Geometry check sheet. Reference: the model listing, model coordinates, mm. A direction names the side the tool comes from. Coordinates: 2 decimals unless noted, no trailing zeros. Loops run counter-clockwise (first coordinate to the right, second up) from the corner with the lowest first, then second, coordinate; pieces in that order, holes last.
Autodesk Inventor part; units mm, degrees
ref_plane "YZ Plane" through (0, 0, 0) normal (1, 0, 0) x (0, 1, 0)
ref_plane "XZ Plane" through (0, 0, 0) normal (0, 1, 0) x (-1, 0, 0)
ref_plane "XY Plane" through (0, 0, 0) normal (0, 0, 1) x (1, 0, 0)
sketch "Boceto2" plane through (0, 0, 0) normal (0, 1, 0) x (-1, 0, 0)
  line L0 (0, 0) -> (100, 0)
  line L1 (100, 0) -> (100, -200)
  line L2 (100, -200) -> (0, -200)
  line L3 (0, -200) -> (0, 0)
  dimension "d2" = 200
  dimension "d3" = 100
extrude "Extrusión1" add sketch "Boceto2" along normal blind 5
sketch "Boceto3" plane through (0, 5, 0) normal (0, 1, 0) x (1, 0, 0)
  line L0 (-100, 200) -> (-100, 0)
  line L1 (-100, 55) -> (-120, 55)
  line L2 (-120, 55) -> (-120, 95)
  line L3 (-120, 95) -> (-100, 95)
  line L4 (-100, 95) -> (-100, 55)
  line L5 (0, 0) -> (0, 200)
  line L6 (0, 55) -> (20, 55)
  line L7 (20, 55) -> (20, 95)
  line L8 (20, 95) -> (0, 95)
  line L9 (0, 95) -> (0, 55)
  line L10 (-100, 0) -> (0, 0)
  circle A0 centre (-110, 75) radius 2.5
  circle A1 centre (10, 75) radius 2.5
  point P0 (0, 95)
  dimension "d6" = 20
  dimension "d7" = 40
  dimension "d8" = 20
  dimension "d9" = 40
  dimension "d10" = 55
  dimension "d11" = 5
  dimension "d12" = 5
extrude "Extrusión2" add sketch "Boceto3" against normal blind 5
thread "Rosca1"
thread "Rosca2"
sketch "Boceto4" plane through (0, 5, 0) normal (0, 1, 0) x (1, 0, 0)
  line L0 (-100, 200) -> (-100, 95)
  line L1 (0, 95) -> (0, 200)
  line L2 (-100, 200) -> (0, 200)
  line L3 (0, 200) -> (0, 190)
  line L4 (0, 190) -> (-100, 190)
  line L5 (-100, 190) -> (-100, 200)
  line L6 (0, 55) -> (-100, 55)
  line L7 (-100, 55) -> (-100, 65)
  line L8 (-100, 65) -> (0, 65)
  line L9 (0, 65) -> (0, 55)
  line L10 (-100, 15) -> (0, 15)
  line L11 (0, 15) -> (0, 25)
  line L12 (0, 25) -> (-100, 25)
  line L13 (-100, 25) -> (-100, 15)
  line L14 (-100, 0) -> (0, 0)
  dimension "d19" = 10
  dimension "d20" = 100
  dimension "d21" = 10
  dimension "d22" = 100
  dimension "d24" = 30
  dimension "d56" = 125
extrude "Extrusión3" add sketch "Boceto4" along normal blind 60
sketch "Boceto5" plane through (0, 0, -200) normal (0, 0, -1) x (-1, 0, 0)
  circle A0 centre (50, 40) radius 5
  line L0 (0, 0) -> (0, 65)
  line L1 (0, 0) -> (100, 0)
  dimension "d28" = 10
  dimension "d29" = 50
  dimension "d34" = 40
extrude "Extrusión4" cut sketch "Boceto5" against normal blind 10
sketch "Boceto6" plane through (0, 5, -65) normal (0, 0, -1) x (-1, 0, 0)
  circle A0 centre (50, 35) radius 5
  circle A1 centre (50, 35) radius 5
  point P0 (0, -5)
extrude "Extrusión5" cut sketch "Boceto6" against normal blind 10
sketch "Boceto7" plane through (-100, 5, -15) normal (0, 0, 1) x (1, 0, 0)
  circle A0 centre (50, 35) radius 5
  circle A1 centre (50, 35) radius 4
  circle A2 centre (36.1091, 50) radius 2.5
  circle A3 centre (63.8909, 50) radius 2.5
  line L0 (0, 0) -> (0, 60)
  line L1 (100, 0) -> (100, 60)
  circle A4 centre (34.6472, 21.5) radius 2.5
  circle A5 centre (65.3528, 21.5) radius 2.5
  line L2 (0, 60) -> (100, 60)
  line L3 (0, 0) -> (100, 0)
  point P0 (100, -5)
  dimension "d35" = 8
  dimension "d36" = 5
  dimension "d37" = 5
  dimension "d41" = 5
  dimension "d42" = 5
  dimension "d45" = 10
  dimension "d47" = 10
  dimension "d50" = 20.444
  dimension "d51" = 28.5
  dimension "d52" = 20.444
  dimension "d53" = 20.444
  dimension "d54" = 20.444
  dimension "d55" = 28.5
extrude "Extrusión6" cut sketch "Boceto7" against normal blind 10 contours A1 | A2 | A3 | A4 | A5
properties part number "Base_motor"
1) Section check D-D on y = 26.5. Record the cut outline in (x, z), and give its area (3 significant figures).
Data:
outline: (-100, -200) - (0, -200) - (0, -190) - (-100, -190) - close; (-100, -65) - (0, -65) - (0, -55) - (-100, -55) - close; (-100, -25) - (-67.85, -25) - (-67.85, -15) - (-100, -15) - close; (-62.85, -25) - (-37.15, -25) - (-37.15, -15) - (-62.85, -15) - close; (-32.15, -25) - (0, -25) - (0, -15) - (-32.15, -15) - close
area: 2,900 mm2
2) Section check C-C on x = 10. Record the cut outline in (y, z).
Data:
outline: (0, -95) - (5, -95) - (5, -77.5) - (0, -77.5) - close; (0, -72.5) - (5, -72.5) - (5, -55) - (0, -55) - close
3) Section check B-B on z = -75. Record the cut outline in (x, y), and give its area (3 significant figures).
Data:
outline: (-120, 0) - (-112.5, 0) - (-112.5, 5) - (-120, 5) - close; (-107.5, 0) - (7.5, 0) - (7.5, 5) - (-107.5, 5) - close; (12.5, 0) - (20, 0) - (20, 5) - (12.5, 5) - close
area: 650 mm2
4) Section check A-A on x = -50. Record the cut outline in (y, z).
Data:
outline: (0, -200) - (35, -200) - (35, -190) - (5, -190) - (5, -65) - (35, -65) - (35, -55) - (5, -55) - (5, -25) - (36, -25) - (36, -15) - (5, -15) - (5, 0) - (0, 0) - close; (44, -25) - (65, -25) - (65, -15) - (44, -15) - close; (45, -200) - (65, -200) - (65, -190) - (45, -190) - close; (45, -65) - (65, -65) - (65, -55) - (45, -55) - close
5) Mould release check, pull along Z, two halves, no side actions. Record for faces 1 (the flat face through (10, 3, -95)), 2 (the cylindrical face through (-62.97, 27.25, -19.93)), 3 (the cylindrical face through (9.46, 2.54, -72.56)): +Z half, -Z half, draft (parallel to the pull), parting line (faces both ways), or undercut.
Data:
face 1: -Z half
face 2: draft
face 3: undercut
6) Access from +Z, -Z, +X, -X, +Y, -Y to the whole of each face (thin tool, end or side, straight path). Record for faces 4 (the flat face through (-49, 35, -25)), 5 (the cylindrical face through (-49.349, 44.957, -60.07)), 6 (the flat face through (-100, 25, -23)).
Data:
face 4: +X, -X, +Y
face 5: -Z
face 6: +Z, -X, +Y, -Y
7) Material ranges on probe 1 along Z at (x, y) = (-31.5, 30); probe 2 along X at (y, z) = (3.7, -75); probe 3 along Z at (x, y) = (-110, 1.5), recorded low to high.
Data:
probe 1: z = -200 to -190, -65 to -55, -25 to -15
probe 2: x = -120 to -112.5, -107.5 to 7.5, 12.5 to 20
probe 3: z = -95 to -77.5, -72.5 to -55
8) Depth check by flat-ended pin: pin 1 (4 mm diameter, centred on x = 14.5, y = 3, fed in from -Z); pin 2 (9 mm diameter, centred on x = -67, z = -42, fed in from +Y); pin 3 (12 mm diameter, centred on y = 52, z = -25.5, fed in from -X); pin 4 (4 mm diameter, centred on x = -95.5, z = -89.5, fed in from -Y). Enter the tip coordinate at first touch or a pass-through.
Data:
pin 1: stops at z = -95
pin 2: stops at y = 5
pin 3: stops at x = -100
pin 4: stops at y = 0
